from build123d import *

# Parameters (mm, degrees)
F2_SIZE  = 0.1
F3_W     = 2.394506
F3_H     = 1.124954
F4_DEPTH = 12.001


with BuildPart() as f1:
    # F0 (on Top) → F1 (revolve)
    with BuildSketch(Plane.XY):
        with BuildLine():
            Line((-6, 0.8), (-6, 0))
            Line((-6, 0), (6, 0))
            Line((6, 0), (6, 0.8))
            Line((6, 0.8), (4, 0.8))
            ThreePointArc((4, 0.8), (3.034511, 0.406031), (2, 0.275))
            Line((2, 0.275), (0, 0.275))
            Line((0, 0.275), (-2, 0.275))
            ThreePointArc((-2, 0.275), (-3.034511, 0.406031), (-4, 0.8))
            Line((-4, 0.8), (-6, 0.8))
        make_face()
    revolve(axis=Axis((0, 0, 0), (1, 0, 0)))

    # F2
    f2_edges = [f1.edges().sort_by_distance(p)[0] for p in [
        (-6, -0.8, 0),
        (6, -0.8, 0),
    ]]
    chamfer(f2_edges, length=F2_SIZE)

    # F3 (on face) → F4 (cut, through all)
    with BuildSketch(Plane(origin=(-6, 0, 0), x_dir=(0, -1, 0), z_dir=(-1, 0, 0))):
        with Locations((-0.261201, 0.562477)):
            Rectangle(F3_W, F3_H)
    extrude(amount=-F4_DEPTH, mode=Mode.SUBTRACT)


solid = f1.part
Build history of the part. All positions in model axes, mm. Give positions to 0.01 mm unless a question says otherwise; leave off trailing zeros. Loops run counter-clockwise (first coordinate to the right, second up) from the corner with the lowest first, then second, coordinate; pieces in that order, holes last. Notation, with made-up numbers: (63.5, 63.25) -> (86.5, 63.25) arc R26 ccw to (86.5, 77.25) -> close; hole circle Ø8 at (14, -19.75). An arc over 180 degrees is marked (long way). Answer in a Markdown table with one row per item.
Item 1: Slice it at C-C on x = -2.75. Write the cut outline in (y, z), plus the area to 3 significant figures.
Findings below:
| item | result |
|---|---|
| outline | (-0.34, 0) arc R0.34 ccw to (0.34, 0) -> close |
| area | 0.184 mm² |
Item 2: Slice it at B-B on x = -4.5. Write the cut outline in (y, z).
Findings below:
| item | result |
|---|---|
| outline | (-0.8, 0) arc R0.8 ccw to (0.8, 0) -> close |
Item 3: Slice it at A-A on y = 0. Write the cut outline in (x, z) (3 decimals), plus the area to 3 significant figures.
Findings below:
| item | result |
|---|---|
| outline | (-6, -0.7) -> (-5.9, -0.8) -> (-4, -0.8) arc R4 cw to (-2, -0.275) -> (2, -0.275) arc R4 cw to (4, -0.8) -> (5.9, -0.8) -> (6, -0.7) -> (6, 0) -> (-6, 0) -> close |
| area | 6.06 mm² |
Item 4: Probe line 1 along Y through (x, z) = (5, -0.05); line 2 along X through (y, z) = (0.55, -0.3); line 3 along X through (y, z) = (-0.45, -0.4). List the from-to ranges inside material, lowest first. Write a range as [from, to].
Findings below:
| item | result |
|---|---|
| line 1 | y = [-0.8, 0.8] |
| line 2 | x = [-6, -3.66], [3.66, 6] |
| line 3 | x = [-6, -3.6], [3.6, 6] |
